from build123d import *

# Parameters (mm, degrees)
SKETCH2_W           = 12.7
SKETCH2_H           = 171.7294
BOSS_EXTRUDE2_DEPTH = 381
CUT_EXTRUDE1_DEPTH  = 13.7
CUT_EXTRUDE2_DEPTH  = 172.7294


with BuildPart() as part:
    # Sketch2 → Boss-Extrude2 (new body)
    with BuildSketch(Plane.XY):
        with Locations((-6.35, 85.8647)):
            Rectangle(SKETCH2_W, SKETCH2_H)
    extrude(amount=BOSS_EXTRUDE2_DEPTH)

    # Sketch3 → Cut-Extrude1 (cut, through all)
    with BuildSketch(Plane(origin=(0, 0, 0), x_dir=(0, 0, -1), z_dir=(1, 0, 0))):
        Polygon((-252.1712, 0), (-298.185954047, 171.7294), (-381, 171.7294), (-381, 0), align=None)
    extrude(amount=-CUT_EXTRUDE1_DEPTH, mode=Mode.SUBTRACT)

    # Sketch4 → Cut-Extrude2 (cut, through all)
    with BuildSketch(Plane(origin=(0, 171.7294, 0), x_dir=(1, 0, 0), z_dir=(0, 1, 0))):
        Polygon((0, 0), (-12.7, -12.7), (-12.7, 0), align=None)
    extrude(amount=-CUT_EXTRUDE2_DEPTH, mode=Mode.SUBTRACT)


solid = part.part
Here's how the part is built. I have some questions about the finished solid (model axes, mm). Round coordinates to 2 decimals unless told otherwise and drop trailing zeros. Write each loop counter-clockwise with the first axis right and the second up, starting at its lowest first coordinate (ties: lowest second). Pieces come first, ordered by that corner, then holes.
1. Suppose I cut it at B-B (y = 52.5). List the corners of the cut face in (x, z) for me.
2. Will these pins go through, and if not, where does the flat tip stop? pin 1 Ø3 at (x, y) = (-9, 152.5) entering from +Z; pin 2 Ø6 at (x, y) = (-3.5, 147) entering from +Z; pin 3 Ø1 at (x, y) = (-3.5, 44.5) entering from -Z.
3. Suppose I cut it at A-A (x = -3). List the corners of the cut face in (y, z) for me.
4. I need wall thicknesses on L1, parallel to Z at x = -1.5, y = 95; L2, parallel to Z at x = -10.75, y = 108. Which ranges of each line are inside material? Lowest first, please.
Answer sheet:
1. outline: (-12.7, 12.7) - (0, 0) - (0, 266.24) - (-12.7, 266.24) - close
2. pin 1: stops at z = 293.44
2. pin 2: stops at z = 292.36
2. pin 3: stops at z = 3
3. outline: (0, 3) - (171.73, 3) - (171.73, 298.19) - (0, 252.17) - close
4. L1: z = 1.5 to 277.63
4. L2: z = 10.75 to 281.11
